Autodesk Fusion 360 part; units mm, degrees
sketch "Esquisse1" plane through (0, 0, 0) normal (0, 0, 1) x (1, 0, 0)
  line L0 (0, 0) -> (85, 0)
  line L1 (85, 0) -> (85, 55)
  line L2 (85, 55) -> (0, 55)
  line L3 (0, 55) -> (0, 0)
  dimension "d1" = 85
  dimension "d2" = 55
sketch "Esquisse2" plane through (0, 0, 0) normal (0, 0, 1) x (1, 0, 0)
  line L0 (-2, -2) -> (87, -2)
  line L1 (87, -2) -> (87, 57)
  line L2 (87, 57) -> (-2, 57)
  line L3 (-2, 57) -> (-2, -2)
  line L4 (0, 0) -> (85, 0)
  line L5 (85, 55) -> (0, 55)
  line L6 (85, 0) -> (85, 55)
  line L7 (0, 55) -> (0, 0)
  line L8 (87.5, -2.5) -> (87.5, 57.5)
  line L9 (87.5, 57.5) -> (-2.5, 57.5)
  line L10 (-2.5, 57.5) -> (-2.5, -2.5)
  line L11 (-2.5, -2.5) -> (87.5, -2.5)
  dimension "d3" = 2
  dimension "d4" = 2
  dimension "d5" = 2
  dimension "d6" = 2
  dimension "d7" = 0.5
extrude "Extrusion1" add sketch "Esquisse2" along normal blind 5 contours L4 L5 L6 L7 makes body 1
extrude "Extrusion2" add sketch "Esquisse2" against normal blind 0.5 separate body contours L0 L1 L2 L3 makes body 2
extrude "Extrusion3" add sketch "Esquisse2" along normal blind 5.5 and the other way blind 0.5 contours L8 L9 L10 L11 bodies 2
extrude "Extrusion4" add 1 faces at (85, 18.3333, -0.1667) along direction (-1, 0, 0) blind 85 on bodies 2 bodies 2
sketch "Esquisse3" plane through (0, 0, 5.5) normal (0, 0, 1) x (-1, 0, 0)
  line L0 (2, 2) -> (2, -57)
  line L1 (2, -57) -> (-87, -57)
  line L2 (-87, -57) -> (-87, 2)
  line L3 (-87, 2) -> (2, 2)
  line L4 (2.5, 2.5) -> (-87.5, 2.5)
  line L5 (-87.5, 2.5) -> (-87.5, -57.5)
  line L6 (-87.5, -57.5) -> (2.5, -57.5)
  line L7 (2.5, -57.5) -> (2.5, 2.5)
  line L8 (2.5, 2.5) -> (-87.5, 2.5)
  line L9 (-87.5, 2.5) -> (-87.5, -57.5)
  line L10 (-87.5, -57.5) -> (2.5, -57.5)
  line L11 (2.5, -57.5) -> (2.5, 2.5)
  dimension "d18" = 60
  dimension "d19" = 90
extrude "Extrusion5" add sketch "Esquisse3" along normal blind 0.5 separate body contours L0 L1 L2 L3 makes body 3
extrude "Extrusion6" add 1 faces at (-2, 17.6667, 5.6667) along direction (-1, 0, 0) blind 0.5 on bodies 3 bodies 3
extrude "Extrusion7" add 1 faces at (27.3333, 57, 5.8333) along direction (0, 1, 0) blind 0.5 on bodies 3 bodies 3
extrude "Extrusion8" add 1 faces at (87, 37.6667, 5.8333) along direction (1, 0, 0) blind 0.5 on bodies 3 bodies 3
extrude "Extrusion9" add 1 faces at (27.5, -2, 5.6667) along direction (0, -1, 0) blind 0.5 on bodies 3 bodies 3
sketch "Esquisse4" plane through (87.5, 0, 0) normal (1, 0, 0) x (0, 1, 0)
  line L0 (57.5, -0.5) -> (57.5, 5.5)
  line L1 (57.5, 5.5) -> (-2.5, 5.5)
  line L2 (-2.5, 5.5) -> (-2.5, -0.5)
  line L3 (-2.5, -0.5) -> (57.5, -0.5)
  line L4 (-2, 0.5) -> (57, 0.5)
  line L5 (57, 0.5) -> (57, 0)
  line L6 (57, 0) -> (-2, 0)
  line L7 (-2, 0) -> (-2, 0.5)
  line L8 (-2.5, -0.5) -> (2.5, -0.5)
  line L9 (2.5, -0.5) -> (2.5, 4.5)
  line L10 (2.5, 4.5) -> (-2.5, 4.5)
  line L11 (-2.5, 4.5) -> (-2.5, -0.5)
  line L12 (57.5, -0.5) -> (52.5, -0.5)
  line L13 (52.5, -0.5) -> (52.5, 4.5)
  line L14 (52.5, 4.5) -> (57.5, 4.5)
  line L15 (57.5, 4.5) -> (57.5, -0.5)
  dimension "d30" = 0.5
  dimension "d31" = 0.5
  dimension "d32" = 0.5
  dimension "d33" = 0.5
  dimension "d34" = 5
  dimension "d35" = 5
  dimension "d36" = 5
  dimension "d37" = 5
extrude "Extrusion10" add sketch "Esquisse4" along normal blind 5 contours L2 L3 L4 L6 L7 L8 L9 L10 L11 bodies 2
extrude "Extrusion11" add sketch "Esquisse4" along normal blind 5 contours L0 L3 L4 L5 L6 L12 L13 L14 L15 bodies 2
extrude "Extrusion12" cut sketch "Esquisse4" against normal blind 1 contours L4 L6 L9 L13 bodies 2
extrude "Extrusion13" cut 1 faces at (87.3333, 2.5, 0.1667) along direction (0, -1, 0) blind 4.5 on bodies 2 bodies 2
extrude "Extrusion14" cut 1 faces at (87.3333, 52.5, 0.1667) along direction (0, 1, 0) blind 4.5 on bodies 2 bodies 2
extrude "Extrusion15" add 1 faces at (89.1667, 0.8333, 4.5) along direction (0, 0, 1) blind 1 on bodies 2 bodies 2
extrude "Extrusion16" add 1 faces at (89.1667, 54.1667, 4.5) along direction (0, 0, 1) blind 1 on bodies 2 bodies 2
extrude "Extrusion17" add 1 faces at (90.8333, 0.8333, 5.5) along direction (0, 0, 1) blind 0.5 on bodies 2 bodies 2
extrude "Extrusion18" add 1 faces at (60.8333, -2.5, 3.8333) along direction (0, -1, 0) blind 0.5 on bodies 2 bodies 2
extrude "Extrusion19" add 1 faces at (-2.5, 17.1667, 3.8333) along direction (-1, 0, 0) blind 0.5 on bodies 2 bodies 2
sketch "Esquisse5" plane through (0, 0, 6) normal (0, 0, 1) x (-1, 0, 0)
  line L0 (2, 2) -> (2, -57)
  line L1 (2, -57) -> (-87, -57)
  line L2 (-87, -57) -> (-87, 2)
  line L3 (-87, 2) -> (2, 2)
  line L4 (-92.5, 3) -> (-92.5, -2.5)
  line L5 (-92.5, -2.5) -> (-87.5, -2.5)
  line L6 (-87.5, -2.5) -> (-87.5, -52.5)
  line L7 (-87.5, -52.5) -> (-92.5, -52.5)
  line L8 (-92.5, -52.5) -> (-92.5, -57.5)
  line L9 (-92.5, -57.5) -> (3, -57.5)
  line L10 (3, -57.5) -> (3, 3)
  line L11 (3, 3) -> (-92.5, 3)
  line L12 (-87.5, 3) -> (3, 3)
  line L13 (3, 3) -> (3, -2.5)
  line L14 (3, -2.5) -> (-87.5, -2.5)
  line L15 (-87.5, -2.5) -> (-87.5, 3)
  line L16 (3, -57.5) -> (-87.5, -57.5)
  line L17 (-87.5, -57.5) -> (-87.5, -52.5)
  line L18 (-87.5, -52.5) -> (3, -52.5)
  line L19 (3, -52.5) -> (3, -57.5)
  dimension "d58" = 5.5
extrude "Extrusion20" add sketch "Esquisse5" along normal blind 0.5 contours L0 L2 L3 L10 L11 L12 L13 L14 L15 | L0 L2 L3 L14 bodies 2
extrude "Extrusion21" add 1 faces at (89.1667, -1.1667, 6) along direction (0, 0, 1) blind 0.5 on bodies 2 bodies 2
extrude "Extrusion22" add sketch "Esquisse5" along normal blind 0.5 contours L0 L1 L2 L9 L10 L16 L17 L18 L19 | L0 L1 L2 L18 bodies 2
extrude "Extrusion23" add sketch "Esquisse5" along normal blind 0.5 contours L7 L8 L9 L17 bodies 2
sketch "Esquisse6" plane through (0, 57.5, 0) normal (0, 1, 0) x (-1, 0, 0)
  line L0 (-92.5, 6.5) -> (-92.5, -0.5)
  line L1 (-92.5, -0.5) -> (3, -0.5)
  line L2 (3, -0.5) -> (3, 6.5)
  line L3 (3, 6.5) -> (-92.5, 6.5)
  line L4 (2.5, 6) -> (-87.5, 6)
  line L5 (-87.5, 6) -> (-87.5, 5.5)
  line L6 (-87.5, 5.5) -> (2.5, 5.5)
  line L7 (2.5, 5.5) -> (2.5, 6)
  dimension "d67" = 90
  dimension "d68" = 0.5
  dimension "d69" = 0.5
  dimension "d70" = 0.5
extrude "Extrusion24" cut sketch "Esquisse6" against normal blind 60 contours L4 L5 L6 L7 bodies 2
hidden bodies 1 3
Source: CAD feature listing. Evaluate the final solid. Frame: model axes, mm. A direction names the side the tool comes from. Round coordinates to 2 decimals unless told otherwise and drop trailing zeros. Loops run counter-clockwise (first coordinate to the right, second up) from the corner with the lowest first, then second, coordinate; pieces in that order, holes last.
Q1. Section A-A, the plane x = 57.5. Return loops of the section in (y, z).
Q2. Section B-B, the plane y = 6. Return loops of the section in (x, z).
Q3. First-contact query: P1, Ø1.5, axis at x = 72, y = 15, coming from the +Z side; P2, Ø1.5, axis at y = 25, z = 2, coming from the +X side. Flat tips, straight axial feed; report the tip coordinate or a pass-through.
Q4. Mould query, pull axis X, two halves, no side actions, for faces 1 (the face through (58.7, 52.5, 6.2)), 2 (the face through (45, -2, 3)), 3 (the face through (-3, 28, 3)). Classes: pulls with the +X half, pulls with the -X half, needs draft (parallel to the pull), parting line crosses it, or undercut.
Q5. Section C-C, the plane z = 2. Return loops of the section in (x, y), plus the area to 3 significant figures.
Q6. Access query for faces 4 (the face through (87.3, 27.4, 0.5)), 5 (the face through (87.5, 27, 3)), 6 (the face through (58.7, 2.5, 6.2)), 7 (the face through (42, 55, 6)), 8 (the face through (-2, 28, 3)). Directions: +Z, -Z, +X, -X, +Y, -Y. A direction counts if a zero-diameter tool reaches every point of the face in a straight line with its end or side. Return the directions, or none.
Q7. Ray query, line 1 (Y direction, x = 79, z = 1.5); line 2 (X direction, y = 38.5, z = 1.5); line 3 (X direction, y = 54.5, z = 1.5). Return the intervals inside material, ascending.
Solutions:
1. outline: (-3, -0.5) - (57.5, -0.5) - (57.5, 5.5) - (57, 5.5) - (57, 0) - (-2, 0) - (-2, 5.5) - (-2.5, 5.5) - (-2.5, 6) - (2.5, 6) - (2.5, 6.5) - (-3, 6.5) - close; (52.5, 6) - (57.5, 6) - (57.5, 6.5) - (52.5, 6.5) - close
2. outline: (-3, -0.5) - (87.5, -0.5) - (87.5, 0) - (-2, 0) - (-2, 5.5) - (-2.5, 5.5) - (-2.5, 6) - (-3, 6) - close; (87, 0.5) - (87.5, 0.5) - (87.5, 5.5) - (87, 5.5) - close
3. P1: stops at z = 0
3. P2: stops at x = 87.5
4. face 1: needs draft
4. face 2: undercut
4. face 3: pulls with the -X half
5. outline: (-3, -3) - (92.5, -3) - (92.5, 2.5) - (87.5, 2.5) - (87.5, 52.5) - (92.5, 52.5) - (92.5, 57.5) - (-3, 57.5) - close; hole (-2, -2) - (87, -2) - (87, 57) - (-2, 57) - close
5. area: 277 mm2
6. face 4: +X
6. face 5: +Z, -Z, +X
6. face 6: +Z, +X
6. face 7: +Y
6. face 8: none
7. line 1: y = -3 to -2, 57 to 57.5
7. line 2: x = -3 to -2, 87 to 87.5
7. line 3: x = -3 to -2, 87 to 92.5
